```python
from build123d import *

# Parameters (mm, degrees)
BOSS_EXTRUDE1_DEPTH             = 3.4036
F_1_4_CLEARANCE_HOLE1_D         = 6.7564
M4_CLEARANCE_HOLE1_D            = 4.5
HOLE_FOR_1_4_300_SC_NUTS_SP_1_D = 8.7376


with BuildPart() as part:
    # Sketch1 → Boss-Extrude1 (new body)
    with BuildSketch(Plane.XY):
        with BuildLine():
            Line((-115.560967743, -45.044749956), (-2.419218956, -16.835343693))
            ThreePointArc((-2.419218956, -16.835343693), (0, -16.538300956), (2.419218956, -16.835343693))
            Line((2.419218956, -16.835343693), (115.560967743, -45.044749956))
            ThreePointArc((115.560967743, -45.044749956), (121.713421794, -49.59732647), (122.84470605, -57.166926175))
            Line((122.84470605, -57.166926175), (115.224166338, -87.731241553))
            ThreePointArc((115.224166338, -87.731241553), (110.671589825, -93.883695604), (103.101990119, -95.014979859))
            Line((103.101990119, -95.014979859), (2.419218956, -69.911945605))
            ThreePointArc((2.419218956, -69.911945605), (0, -69.614902867), (-2.419218956, -69.911945605))
            Line((-2.419218956, -69.911945605), (-103.101990119, -95.014979859))
            ThreePointArc((-103.101990119, -95.014979859), (-110.671589825, -93.883695604), (-115.224166338, -87.731241553))
            Line((-115.224166338, -87.731241553), (-122.84470605, -57.166926175))
            ThreePointArc((-122.84470605, -57.166926175), (-121.713421794, -49.59732647), (-115.560967743, -45.044749956))
        make_face()
    extrude(amount=-BOSS_EXTRUDE1_DEPTH)

    # 1/4 Clearance Hole1 (through all)
    with Locations(Plane.XY):
        with Locations((-74.335136024, -53.317040996), (74.335136024, -53.317040996)):
            Hole(F_1_4_CLEARANCE_HOLE1_D / 2)

    # M4 Clearance Hole1 (through all)
    with Locations(Plane.XY):
        with Locations((-110.721225759, -62.389112081), (-37.949046288, -44.244969911), (37.949046288, -44.244969911), (110.721225759, -62.389112081)):
            Hole(M4_CLEARANCE_HOLE1_D / 2)

    # Hole for 1/4 300® SC Nuts (SP)1 (through all)
    with Locations(Plane.XY):
        with Locations((-4.6482, -60.701560235), (-4.6482, -28.951560235)):
            Hole(HOLE_FOR_1_4_300_SC_NUTS_SP_1_D / 2)


solid = part.part
```
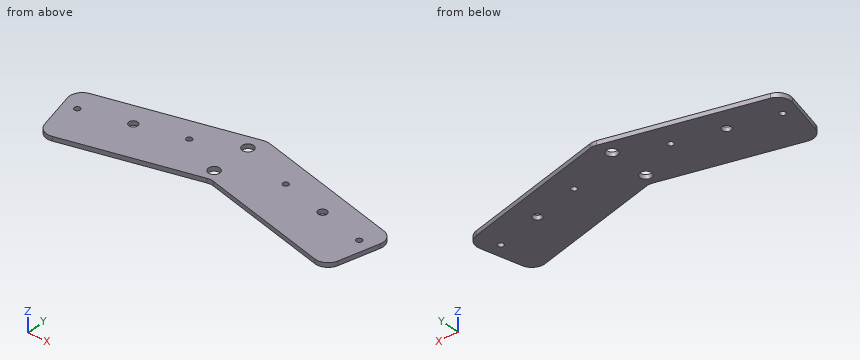
Geometry check sheet. Reference: the model listing, model coordinates, mm. Give positions to 0.01 mm unless a question says otherwise; leave off trailing zeros. Order: outer loops, then holes, each group sorted by start corner. A loop starts at its lowest first (then second) coordinate and runs counter-clockwise, first axis right, second up. Notation, with made-up numbers: (21.5, 73) - (34.5, 73) arc R18 cw to (34.5, 82) - close; hole circle Ø1 at (71.25, -37.75). An arc over 180 degrees is marked (long way). Answer in a Markdown table with one row per item. Add a question column.
Q1. Cross-section at B-B, the plane z = -2.5. Count the separate pieces of the cut face and the enclosed holes in it, then the cut area to 3 significant figures.
Q2. Gauge pin test, flat end, axial feed: pin 1 (8 mm diameter, centred on x = 37, y = -63.5, fed in from +Z). Record the tip position at first contact, or that the pin passes through.
Q3. Cross-section at C-C, the plane x = 88. Enter the section's corners in (y, z), then the cut area to 3 significant figures.
Q4. Cross-section at A-A, the plane y = -76. Enter the section's corners in (x, z), then the cut area to 3 significant figures.
Q5. Material ranges on probe 1 along Y at (x, z) = (-1.5, -3.25); probe 2 along X at (y, z) = (-61, -1.05); probe 3 along X at (y, z) = (-63, -1.5), recorded low to high. Write a range as from..to.
Check values:
| question | item | result |
|---|---|---|
| 1 | separate pieces | 1 |
| 1 | enclosed holes | 8 |
| 1 | area | 12,300 mm^2 |
| 2 | pin 1 | stops at z = 0 |
| 3 | outline | (-91.25, -3.4) - (-38.17, -3.4) - (-38.17, 0) - (-91.25, 0) - close |
| 3 | area | 181 mm^2 |
| 4 | outline | (-118.15, -3.4) - (-26.84, -3.4) - (-26.84, 0) - (-118.15, 0) - close; (26.84, -3.4) - (118.15, -3.4) - (118.15, 0) - (26.84, 0) - close |
| 4 | area | 622 mm^2 |
| 5 | probe 1 | y = -69.73..-63.73, -57.67..-31.98, -25.92..-16.65 |
| 5 | probe 2 | x = -121.89..-112.49, -108.95..-9.01, -0.29..108.95, 112.49..121.89 |
| 5 | probe 3 | x = -121.39..-112.89, -108.56..-8.36, -0.93..108.56, 112.89..121.39 |
